```python
from build123d import *

# Parameters (mm, degrees)
F1_DEPTH = 63.5
F0_W     = 25.4
F0_H     = 19.05
F2_DEPTH = 25.4
F3_DEPTH = 7.9375
F4_R     = 6.35


with BuildPart() as f1:
    # F0 (on Front) → F1 (new body, symmetric)
    with BuildSketch(Plane.XZ):
        Polygon((22.225, 19.05), (-41.275, 19.05), (-41.275, 0), (41.275, 0), (41.275, 19.05), align=None)
    extrude(amount=F1_DEPTH, both=True)

    # F0 (on Front) → F2 (join, symmetric)
    with BuildSketch(Plane.XZ):
        with BuildLine():
            Line((22.225, 36.5252), (22.225, 19.05))
            Line((22.225, 19.05), (41.275, 19.05))
            Line((41.275, 19.05), (41.275, 36.5252))
            ThreePointArc((41.275, 36.5252), (45.9246798487, 47.7505201513), (57.15, 52.4002))
            Line((57.15, 52.4002), (60.325, 52.4002))
            Line((60.325, 52.4002), (60.325, 71.4502))
            Line((60.325, 71.4502), (57.15, 71.4502))
            add(Edge.make_bspline(
                [(48.5295077418, 70.3695900555), (51.7256176112, 70.8797706122), (54.6303264693, 71.2419617034), (57.15, 71.4502)],
                knots=[101.0999691386, 101.0999691386, 101.0999691386, 101.0999691386, 111.5045361635, 111.5045361635, 111.5045361635, 111.5045361635], degree=3))
            ThreePointArc((48.5295077418, 70.3695900555), (29.5744100959, 57.9574762777), (22.225, 36.5252))
        make_face()
        with Locations((73.025, 61.9252)):
            Rectangle(F0_W, F0_H)
    extrude(amount=F2_DEPTH, both=True)

    # F0 (on Front) → F3 (join, symmetric)
    with BuildSketch(Plane.XZ):
        with BuildLine():
            add(Edge.make_bspline(
                [(-41.275, 19.05), (-41.096400475, 46.4820152223), (17.4732794163, 65.4122248504), (48.5295077418, 70.3695900555)],
                knots=[0, 0, 0, 0, 101.0999691386, 101.0999691386, 101.0999691386, 101.0999691386], degree=3))
            Line((-41.275, 19.05), (22.225, 19.05))
            Line((22.225, 19.05), (22.225, 36.5252))
            ThreePointArc((22.225, 36.5252), (29.5744100959, 57.9574762777), (48.5295077418, 70.3695900555))
        make_face()
    extrude(amount=F3_DEPTH, both=True)

    # F4
    f4_edges = [f1.edges().sort_by_distance(p)[0] for p in [
        (41.275, -63.5, 9.525),
        (-41.275, -63.5, 9.525),
        (-41.275, 63.5, 9.525),
        (41.275, 63.5, 9.525),
    ]]
    fillet(f4_edges, radius=F4_R)

    # F0 (on Front) → F5 (revolve)
    with BuildSketch(Plane.XZ):
        Polygon((85.725, 76.2), (85.725, 71.4502), (85.725, 52.4002), (85.725, 47.625), (111.125, 47.625), (111.125, 76.2), align=None)
    revolve(axis=Axis((85.725, 0, 61.9125), (0, 0, -1)))


solid = f1.part
```
Can you work these out from the model? Positions are in its coordinate system, mm. A direction names the side the tool comes from. Coordinates: 2 decimals unless noted, no trailing zeros. Loops run counter-clockwise (first coordinate to the right, second up) from the corner with the lowest first, then second, coordinate; pieces in that order, holes last.
1) Imagine slicing it at A-A on z = 10. List the corners of the cut face in (x, y) for me (3 decimals).
2) Thinking about a two-plate mould opening in X: for faces 1 (the cylindrical face through (-39.464, -61.59, 9.392)), 2 (the flat face through (60, 2, 52.4)), 3 (the cylindrical face through (39.365, -61.689, 9.658)), which applies, pulls with the +X half, pulls with the -X half, needs draft (parallel to the pull), parting line crosses it, or undercut?
3) Imagine slicing it at B-B on x = 80. List the corners of the cut face in (y, z) for me (3 decimals).
4) Imagine slicing it at D-D on x = 63.5. List the corners of the cut face in (y, z) for me (3 decimals).
5) Which directions (+Z, -Z, +X, -X, +Y, -Y) give clear straight access to the entire face, cutting with the end or side of a thin tool? Please do faces 4 (the cylindrical face through (45.802, -0.356, 47.626)), 5 (the flat face through (22.225, -17, 28)), 6 (the flat face through (22.225, 17, 28)).
6) Imagine slicing it at C-C on y = -34.5. List the corners of the cut face in (x, z) for me (3 decimals), plus the area to 3 significant figures.
7) I need wall thicknesses on probe 1 along Z at (x, y) = (96, -7) (3 decimals); probe 2 along X at (y, z) = (46, 19) (3 decimals); probe 3 along Y at (x, z) = (-21, 35). Which ranges of each line are inside material? Lowest first, please.
8) For pin 1 (8 mm diameter, centred on y = -2.5, z = 25.5, fed in from -X); pin 2 (16.5 mm diameter, centred on x = -20, y = -35.5, fed in from +Z); pin 3 (6 mm diameter, centred on x = 87, y = -28.5, fed in from -Z); pin 4 (14.5 mm diameter, centred on x = 73, y = 0.5, fed in from -Z) (3 decimals), each with a flat end and sliding along its axis, tell me the tip position at first contact or that it passes through.
Completed:
1. outline: (-41.275, -57.15) arc R6.35 ccw to (-34.925, -63.5) - (34.925, -63.5) arc R6.35 ccw to (41.275, -57.15) - (41.275, 57.15) arc R6.35 ccw to (34.925, 63.5) - (-34.925, 63.5) arc R6.35 ccw to (-41.275, 57.15) - close
2. face 1: pulls with the -X half
2. face 2: undercut
2. face 3: pulls with the +X half
3. outline: (-25.4, 52.4) - (-24.746, 52.4) - (-24.746, 47.625) - (24.746, 47.625) - (24.746, 52.4) - (25.4, 52.4) - (25.4, 71.45) - (24.746, 71.45) - (24.746, 76.2) - (-24.746, 76.2) - (-24.746, 71.45) - (-25.4, 71.45) - close
4. outline: (-25.4, 52.4) - (-12.297, 52.4) - (-12.297, 47.625) - (12.297, 47.625) - (12.297, 52.4) - (25.4, 52.4) - (25.4, 71.45) - (12.297, 71.45) - (12.297, 76.2) - (-12.297, 76.2) - (-12.297, 71.45) - (-25.4, 71.45) - close
5. face 4: -Z, +Y, -Y
5. face 5: +Z, -X, -Y
5. face 6: +Z, -X, +Y
6. outline: (-41.275, 0) - (41.275, 0) - (41.275, 19.05) - (-41.275, 19.05) - close
6. area: 1,570 mm2
7. probe 1: z = 47.625 to 76.2
7. probe 2: x = -41.275 to 41.275
7. probe 3: y = -7.94 to 7.94
8. pin 1: stops at x = -41.1
8. pin 2: stops at z = 19.05
8. pin 3: passes through
8. pin 4: stops at z = 47.625
